Input: dimensioned drawing with shaded views. Units: mm. Origin: part minimum x, y, z. A direction names the side the tool comes from. Coordinates: 2 decimals unless noted, no trailing zeros. Order: outer loops, then holes, each group sorted by start corner. A loop starts at its lowest first (then second) coordinate and runs counter-clockwise, first axis right, second up. Notation, with made-up numbers: (86.5, 47) - (131.5, 47) arc R20 cw to (131.5, 72) - close; hole circle Ø11 at (-28, 44.25). An arc over 180 degrees is marked (long way). Use one line per item in the form item = value. Start each with the question number.
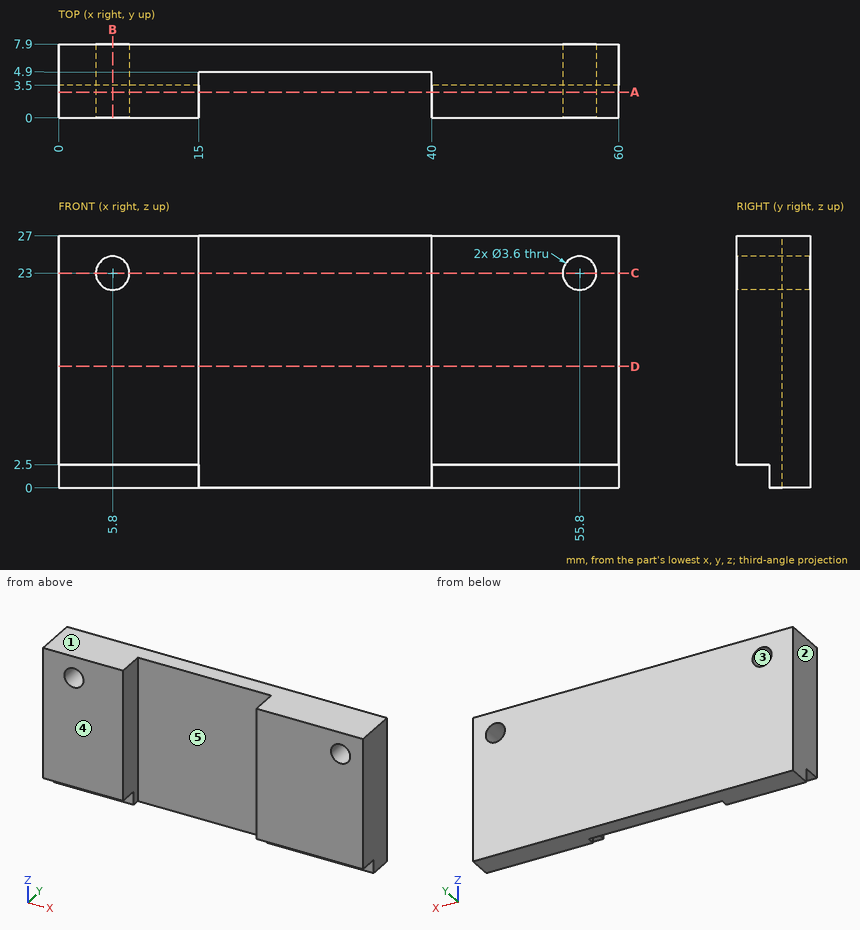
(1) Cut plane D-D on z = 13. Return the cut outline in (x, y).
(2) Cut plane B-B on x = 5.8. Return the cut outline in (y, z).
(3) Cut plane C-C on z = 23. Return the cut outline in (x, y), plus the area to 3 significant figures.
(4) Contact query for flat-ended pins moving along their axis: pin 1 Ø7.5 at (x, z) = (25.5, 14) entering from -Y; pin 2 Ø0.8 at (x, z) = (49.5, 1) entering from -Y; pin 3 Ø1.8 at (x, y) = (52.5, 2) entering from -Z. Output: stop coordinate, or through.
(5) Draft query along Z for the marked faces 1, 2 and 3. Return one class per face: released by +Z, released by -Z, zero draft, split by the parting line, or undercut.
(6) Material intervals for L1, parallel to X at y = 3.25, z = 23; L2, parallel to X at y = 5.5, z = 23; L3, parallel to X at y = 1, z = 14.5, sorted ascending. Write a range as from..to.
(7) Cut plane A-A on y = 2.75. Return the cut outline in (x, z).
(8) Set-up query: the marked faces 4 and 5. Return all of +Z, -Z, +X, -X, +Y, -Y with unobstructed straight access to the full face (end or side cutting, diameter ignored); none if empty.
Check sheet entries:
q1.outline = (0, 0) - (15, 0) - (15, 4.9) - (40, 4.9) - (40, 0) - (60, 0) - (60, 7.9) - (0, 7.9) - close
q2.outline = (0, 2.5) - (3.5, 2.5) - (3.5, 0) - (7.9, 0) - (7.9, 21.2) - (0, 21.2) - close; (0, 24.8) - (7.9, 24.8) - (7.9, 27) - (0, 27) - close
q3.outline = (0, 0) - (4, 0) - (4, 7.9) - (0, 7.9) - close; (7.6, 0) - (15, 0) - (15, 4.9) - (40, 4.9) - (40, 0) - (54, 0) - (54, 7.9) - (7.6, 7.9) - close; (57.6, 0) - (60, 0) - (60, 7.9) - (57.6, 7.9) - close
q3.area = 295 mm^2
q4.pin_1 = 4.9
q4.pin_2 = 3.5
q4.pin_3 = 2.5
q5.face_1 = released by +Z
q5.face_2 = zero draft
q5.face_3 = undercut
q6.L1 = 0..4, 7.6..15, 40..54, 57.6..60
q6.L2 = 0..4, 7.6..54, 57.6..60
q6.L3 = 0..15, 40..60
q7.outline = (0, 2.5) - (15, 2.5) - (15, 27) - (0, 27) - close; (40, 2.5) - (60, 2.5) - (60, 27) - (40, 27) - close; hole circle Ø3.6 at (5.8, 23); hole circle Ø3.6 at (55.8, 23)
q8.face_4 = +Z, -Z, +X, -X, -Y
q8.face_5 = +Z, -Z, -Y
